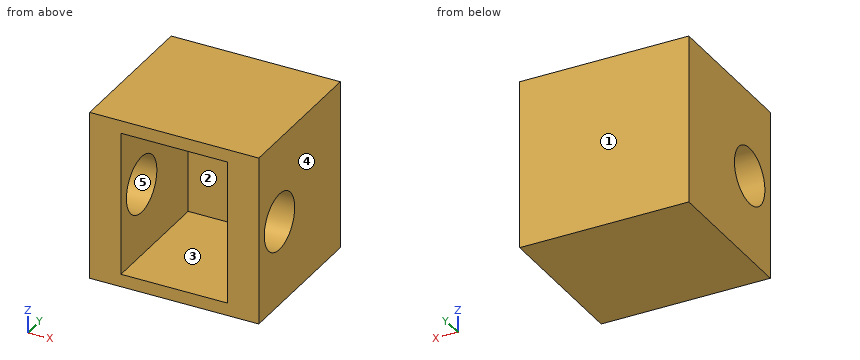
```python
from build123d import *

# Parameters (mm, degrees)
BOSS_EXTRUDE1_DEPTH = 10.795
SKETCH2_R           = 2.12471
CUT_EXTRUDE1_DEPTH  = 13.7
SKETCH3_W           = 10.795
SKETCH3_H           = 0.6985
CUT_EXTRUDE2_DEPTH  = 13.7
SKETCH4_W           = 0.9525
SKETCH4_H           = 11.38936
BOSS_EXTRUDE2_DEPTH = 12.7


with BuildPart() as part:
    # Sketch1 → Boss-Extrude1 (new body)
    with BuildSketch(Plane.XY):
        Polygon((0, 0), (0, 10.08888), (8.001, 10.08888), (8.001, 0), (10.3505, 0), (10.3505, 12.08786), (-2.3495, 12.08786), (-2.3495, 0), align=None)
    extrude(amount=BOSS_EXTRUDE1_DEPTH)

    # Sketch2 → Cut-Extrude1 (cut, through all)
    with BuildSketch(Plane(origin=(10.3505, 0, 0), x_dir=(0, 0, -1), z_dir=(1, 0, 0))):
        with Locations((-5.3975, 3.58648)):
            Circle(SKETCH2_R)
    extrude(amount=-CUT_EXTRUDE1_DEPTH, mode=Mode.SUBTRACT)

    # Sketch3 → Cut-Extrude2 (cut, through all)
    with BuildSketch(Plane(origin=(10.3505, 0, 0), x_dir=(0, 0, -1), z_dir=(1, 0, 0))):
        with Locations((-5.3975, 0.34925)):
            Rectangle(SKETCH3_W, SKETCH3_H)
    extrude(amount=-CUT_EXTRUDE2_DEPTH, mode=Mode.SUBTRACT)

    # Sketch4 → Boss-Extrude2 (add)
    with BuildSketch(Plane(origin=(10.3505, 0, 0), x_dir=(0, 0, -1), z_dir=(1, 0, 0))):
        with Locations((-11.27125, 6.39318)):
            Rectangle(SKETCH4_W, SKETCH4_H)
        with Locations((0.47625, 6.39318)):
            Rectangle(SKETCH4_W, SKETCH4_H)
    extrude(amount=-BOSS_EXTRUDE2_DEPTH)


solid = part.part
```
The listing builds one solid part. Answer for the finished solid, in the listing's coordinates (mm). Face numbers are marked on the shaded views. A direction names the side the tool comes from. Round coordinates to 2 decimals unless told otherwise and drop trailing zeros. Loops run counter-clockwise (first coordinate to the right, second up) from the corner with the lowest first, then second, coordinate; pieces in that order, holes last. Notation, with made-up numbers: (44, 59) -> (57, 59) arc R18 ccw to (57, 90) -> close; hole circle Ø6 at (71.25, -30). An arc over 180 degrees is marked (long way). Use one line per item in the form item = value.
1. The part is cut by section A-A on y = 9. Determine the outline of the cut face in (x, z) (1 decimal).
Answer key:
outline = (-2.3, -1) -> (10.4, -1) -> (10.4, 11.7) -> (-2.3, 11.7) -> close; hole (0, 0) -> (8, 0) -> (8, 10.8) -> (0, 10.8) -> close
2. The part is cut by section B-B on z = 9.5. Determine the outline of the cut face in (x, y).
Answer key:
outline = (-2.35, 0.7) -> (0, 0.7) -> (0, 10.09) -> (8, 10.09) -> (8, 0.7) -> (10.35, 0.7) -> (10.35, 12.09) -> (-2.35, 12.09) -> close
3. Find the intervals of material crossed by probe 1 along Z at (x, y) = (2.75, 9.75) (1 decimal); probe 2 along X at (y, z) = (7.5, 1); probe 3 along Z at (x, y) = (-0.5, 5.5), in increasing order. Write a range as [from, to].
Answer key:
probe_1 = [-1, 0], [10.8, 11.7]
probe_2 = [-2.35, 0], [8, 10.35]
probe_3 = [-0.95, 4.47], [6.32, 11.75]
4. The part is cut by section D-D on z = 6.25. Determine the outline of the cut face in (x, y), and give its area (3 significant figures).
Answer key:
outline = (-2.35, 0.7) -> (0, 0.7) -> (0, 1.64) -> (-2.35, 1.64) -> close; (-2.35, 5.53) -> (0, 5.53) -> (0, 10.09) -> (8, 10.09) -> (8, 5.53) -> (10.35, 5.53) -> (10.35, 12.09) -> (-2.35, 12.09) -> close; (8, 0.7) -> (10.35, 0.7) -> (10.35, 1.64) -> (8, 1.64) -> close
area = 51.2 mm²
5. A tool of negligible diameter and unlimited length cuts with its end or side. For the marked faces 1 and 2, from which of +Z, -Z, +X, -X, +Y, -Y can it reach the whole face along a straight path? Write none if from no direction.
Answer key:
face_1 = +Z, -Z, +X, -X, +Y
face_2 = -Y
6. The part is cut by section C-C on x = 1. Determine the outline of the cut face in (y, z) (1 decimal), and give its area (3 significant figures).
Answer key:
outline = (0.7, -1) -> (12.1, -1) -> (12.1, 11.7) -> (0.7, 11.7) -> (0.7, 10.8) -> (10.1, 10.8) -> (10.1, 0) -> (0.7, 0) -> close
area = 43.3 mm²
7. For a pull along X with two mould halves and no side action, classify the marked faces 3, 4 and 5 as released by +X, released by -X, zero draft, split by the parting line, or undercut.
Answer key:
face_3 = undercut
face_4 = released by +X
face_5 = zero draft
